from build123d import *

# Parameters (mm, degrees)
SKETCH1_R                     = 12.6492
BOSS_EXTRUDE1_DEPTH           = 2.4384
F_8_THREADED_ROD_CLEARANCE_D  = 4.4958
EJECTION_CHARGE_PASSTHROUGH_D = 2.7051


with BuildPart() as part:
    # Sketch1 → Boss-Extrude1 (new body)
    with BuildSketch(Plane(origin=(0, 0, 0), x_dir=(0, 0, -1), z_dir=(1, 0, 0))):
        Circle(SKETCH1_R)
    extrude(amount=BOSS_EXTRUDE1_DEPTH)

    # #8 Threaded Rod Clearance (through all)
    with Locations(Plane(origin=(2.4384, 0, 0), x_dir=(0, 0, -1), z_dir=(1, 0, 0))):
        with Locations((0, 0)):
            Hole(F_8_THREADED_ROD_CLEARANCE_D / 2)

    # Ejection Charge Passthrough (through all)
    with Locations(Plane(origin=(2.4384, 0, 0), x_dir=(0, 0, -1), z_dir=(1, 0, 0))):
        with Locations((-7.9375, 0), (7.9375, 0)):
            Hole(EJECTION_CHARGE_PASSTHROUGH_D / 2)


solid = part.part
Part model, mm, in its own coordinate system. Round coordinates to 2 decimals unless told otherwise and drop trailing zeros. Write each loop counter-clockwise with the first axis right and the second up, starting at its lowest first coordinate (ties: lowest second). Pieces come first, ordered by that corner, then holes. Notation, with made-up numbers: M 64.5,80 L 70.5,80 A25 ccw 70.5,116 Z; hole C 64.5,-23 d9. An arc over 180 degrees is marked long. Return JSON: item names as keys, results as strings. Group by question number.
(1) Two-plate mould, pull along Y, no slides. Class faces 1 (the face through (1.202, 0.406, 9.228)), 2 (the face through (2.438, -3, 0)), 3 (the face through (1, 4, -12)): +Y half, -Y half, draft (parallel to the pull), parting line (faces both ways), or undercut.
(2) Saw through at B-B on z = 0. Write the cut outline in (x, y), then the cut area to 3 significant figures.
(3) Drill centre lines: probe 1 along Y at (x, z) = (1.8, 0); probe 2 along Y at (x, z) = (0.4, -9); probe 3 along Z at (x, y) = (2.1, -0.5). Where is each one in solid material? Low to high.
(4) Saw through at D-D on z = -10.5. Write the cut outline in (x, y), then the cut area to 3 significant figures.
(5) Saw through at A-A on y = 0. Write the cut outline in (x, z), then the cut area to 3 significant figures.
(6) Pin check, flat tip, straight feed: pin 1 Ø2 at (y, z) = (0, -7.94) entering from -X (1 decimal). Stop position of the tip, or through.
(7) Saw through at C-C on x = 0.55. Write the cut outline in (y, z).
Returned:
{
 "1": {"face 1": "undercut", "face 2": "draft", "face 3": "parting line"},
 "2": {"outline": "M 0,-12.65 L 2.44,-12.65 L 2.44,-2.25 L 0,-2.25 Z; M 0,2.25 L 2.44,2.25 L 2.44,12.65 L 0,12.65 Z", "area": "50.7 mm²"},
 "3": {"probe 1": "-12.65 to -2.25, 2.25 to 12.65", "probe 2": "-8.89 to -0.84, 0.84 to 8.89", "probe 3": "-12.64 to -9.19, -6.68 to -2.19, 2.19 to 6.68, 9.19 to 12.64"},
 "4": {"outline": "M 0,-7.05 L 2.44,-7.05 L 2.44,7.05 L 0,7.05 Z", "area": "34.4 mm²"},
 "5": {"outline": "M 0,-12.65 L 2.44,-12.65 L 2.44,-9.29 L 0,-9.29 Z; M 0,-6.58 L 2.44,-6.58 L 2.44,-2.25 L 0,-2.25 Z; M 0,2.25 L 2.44,2.25 L 2.44,6.58 L 0,6.58 Z; M 0,9.29 L 2.44,9.29 L 2.44,12.65 L 0,12.65 Z", "area": "37.5 mm²"},
 "6": {"pin 1": "through"},
 "7": {"outline": "C 0,0 d25.3; hole C 0,0 d4.5; hole C 0,-7.94 d2.71; hole C 0,7.94 d2.71"}
}
